```python
from build123d import *

# Parameters (mm, degrees)
SKETCH1_R           = 8.334375
SKETCH1_W           = 6.477
SKETCH1_H           = 6.477
BOSS_EXTRUDE1_DEPTH = 0.79375
SKETCH2_W           = 6.477
SKETCH2_H           = 6.477
BOSS_EXTRUDE2_DEPTH = 6.35
SKETCH3_R           = 5.1435
CUT_EXTRUDE1_DEPTH  = 1.27
FILLET1_R           = 1.5875
FILLET2_R           = 0.396875
SKETCH5_R           = 5.1435
SKETCH5_W           = 6.477
SKETCH5_H           = 6.477
BOSS_EXTRUDE3_DEPTH = 1.27
BOSS_EXTRUDE4_START = 1.27
SKETCH6_R           = 5.1435
SKETCH6_W           = 6.477
SKETCH6_H           = 6.477
BOSS_EXTRUDE4_DEPTH = 1.27


with BuildPart() as part:
    # Sketch1 → Boss-Extrude1 (new body)
    with BuildSketch(Plane.XY):
        Circle(SKETCH1_R)
        Rectangle(SKETCH1_W, SKETCH1_H, mode=Mode.SUBTRACT)
    extrude(amount=BOSS_EXTRUDE1_DEPTH)

    # Sketch2 → Boss-Extrude2 (add)
    with BuildSketch(Plane.XY.offset(0.79375)):
        Polygon((7.332348419, 0), (3.666174209, 6.35), (-3.666174209, 6.35), (-7.332348419, 0), (-3.666174209, -6.35), (3.666174209, -6.35), align=None)
        Rectangle(SKETCH2_W, SKETCH2_H, mode=Mode.SUBTRACT)
    extrude(amount=BOSS_EXTRUDE2_DEPTH)

    # Sketch3 → Cut-Extrude1 (cut)
    with BuildSketch(Plane(origin=(0, 0, 0), x_dir=(-1, 0, 0), z_dir=(0, 0, -1))):
        Circle(SKETCH3_R)
    extrude(amount=-CUT_EXTRUDE1_DEPTH, mode=Mode.SUBTRACT)

    # Fillet1
    fillet1_edges = [part.edges().sort_by_distance(p)[0] for p in [
        (3.666174209, -6.35, 3.96875),
        (7.332348419, 0, 3.96875),
        (3.666174209, 6.35, 3.96875),
        (-3.666174209, 6.35, 3.96875),
        (-7.332348419, 0, 3.96875),
        (-3.666174209, -6.35, 3.96875),
    ]]
    fillet(fillet1_edges, radius=FILLET1_R)

    # Fillet2
    fillet2_edges = [part.edges().sort_by_distance(p)[0] for p in [
        (-8.334375, 0, 0),
    ]]
    fillet(fillet2_edges, radius=FILLET2_R)

    # Mirror1: part across plane


with BuildPart() as part_1:
    add(part.part)
    add(part.part.mirror(Plane.XY.offset(7.14375)))

    # Sketch5 → Boss-Extrude3 (add)
    with BuildSketch(Plane(origin=(0, 0, 1.27), x_dir=(-1, 0, 0), z_dir=(0, 0, -1))):
        Circle(SKETCH5_R)
        Rectangle(SKETCH5_W, SKETCH5_H, mode=Mode.SUBTRACT)
    extrude(amount=BOSS_EXTRUDE3_DEPTH)

    # Sketch6 → Boss-Extrude4 (add)
    with BuildSketch(Plane.XY.offset(13.0175).offset(BOSS_EXTRUDE4_START)):
        Circle(SKETCH6_R)
        Rectangle(SKETCH6_W, SKETCH6_H, mode=Mode.SUBTRACT)
    extrude(amount=-BOSS_EXTRUDE4_DEPTH)


solid = part_1.part
```
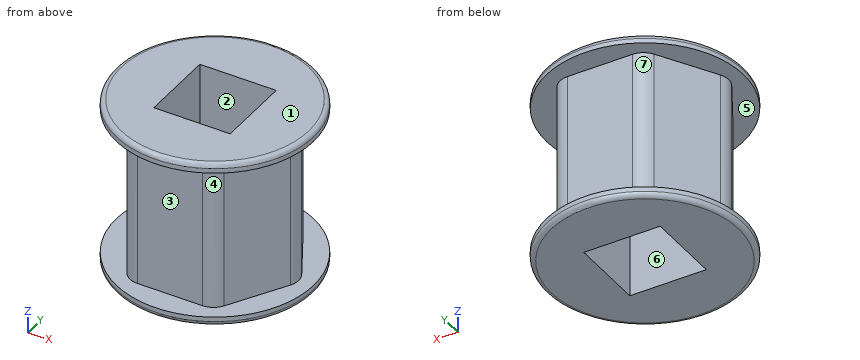
Could you check a few things on this model? Use its own coordinates, in mm. Face numbers are marked on the shaded views. A direction names the side the tool comes from. Give positions to 0.01 mm unless a question says otherwise; leave off trailing zeros. Order: outer loops, then holes, each group sorted by start corner. A loop starts at its lowest first (then second) coordinate and runs counter-clockwise, first axis right, second up.
Q1. Suppose I cut it at A-A, the plane x = 0. Write out the boundary of the cut face in (y, z).
Q2. Suppose I cut it at B-B, the plane y = 0. Write out the boundary of the cut face in (x, z).
Q3. If I drill on line 1 along Y through (x, z) = (-2, 7.5); line 2 along Z through (x, y) = (-6, -5.5); line 3 along X through (y, z) = (3, 13.25), over which ranges is the centre line in solid material (lowest first)?
Q4. I'm going to push flat-ended pins straight in: P1, Ø7, axis at x = -0.5, z = 5.5, coming from the -Y side; P2, Ø1.9, axis at y = 0, z = 7.5, coming from the -X side; P3, Ø4, axis at y = 4, z = 3, coming from the +X side; P4, Ø1.5, axis at x = 1.5, y = -2, coming from the +Z side. Where does each tip first touch, or does it pass through?
Q5. For the marked faces 4, 5, 6 and 7, which set-ups out of +Z, -Z, +X, -X, +Y, -Y let a thin tool reach every point of the face, with its end or its side?
Q6. We'd pull the mould along Y, two halves only. Please class the marked faces 1, 2 and 3: +Y half, -Y half, draft (parallel to the pull), parting line (faces both ways), or undercut.
Solution:
1. outline: (-8.33, 0.4) arc R0.4 ccw to (-7.94, 0) - (-3.24, 0) - (-3.24, 14.29) - (-7.94, 14.29) arc R0.4 ccw to (-8.33, 13.89) - (-8.33, 13.49) - (-6.35, 13.49) - (-6.35, 0.79) - (-8.33, 0.79) - close; (3.24, 0) - (7.94, 0) arc R0.4 ccw to (8.33, 0.4) - (8.33, 0.79) - (6.35, 0.79) - (6.35, 13.49) - (8.33, 13.49) - (8.33, 13.89) arc R0.4 ccw to (7.94, 14.29) - (3.24, 14.29) - close
2. outline: (-8.33, 0.4) arc R0.4 ccw to (-7.94, 0) - (-3.24, 0) - (-3.24, 14.29) - (-7.94, 14.29) arc R0.4 ccw to (-8.33, 13.89) - (-8.33, 13.49) - (-7.09, 13.49) - (-7.09, 0.79) - (-8.33, 0.79) - close; (3.24, 0) - (7.94, 0) arc R0.4 ccw to (8.33, 0.4) - (8.33, 0.79) - (7.09, 0.79) - (7.09, 13.49) - (8.33, 13.49) - (8.33, 13.89) arc R0.4 ccw to (7.94, 14.29) - (3.24, 14.29) - close
3. line 1: y = -6.35 to -3.24, 3.24 to 6.35
3. line 2: z = 0.06 to 0.79, 13.49 to 14.23
3. line 3: x = -5.6 to -3.24, 3.24 to 5.6
4. P1: stops at y = -6.35
4. P2: stops at x = -7.09
4. P3: stops at x = 6.18
4. P4: passes through
5. face 4: +X, -Y
5. face 5: none
5. face 6: +Z, -Z
5. face 7: -X, +Y
6. face 1: draft
6. face 2: undercut
6. face 3: -Y half
